```python
from build123d import *

# Parameters (mm, degrees)
SKETCH1_R               = 2.54
BOSS_EXTRUDE1_DEPTH     = 6.35
SKETCH2_R               = 2.54
BOSS_EXTRUDE2_DEPTH     = 6.35
CUT_EXTRUDE3_DEPTH      = 191.722024651
BOSS_EXTRUDE3_START     = -6.35
BOSS_EXTRUDE3_OUTLINE_R = 2.54
BOSS_EXTRUDE3_DEPTH     = 6.35


# Read off the part's stored shape, not the designer's step: Boss-Extrude3
with BuildPart() as part:
    # Sketch1 → Boss-Extrude1 (new body)
    with BuildSketch(Plane(origin=(0, 0, 0), x_dir=(0, 0, -1), z_dir=(1, 0, 0))):
        with BuildLine():
            Line((-44.569856196, 7.632792855), (2.7669164, -12.394925318))
            ThreePointArc((2.7669164, -12.394925318), (12.623500932, 1.391842028), (0, 12.7))
            ThreePointArc((0, 12.7), (-15.936201096, 21.312567622), (-17.462784388, 39.362730221))
            ThreePointArc((-17.462784388, 39.362730221), (-5.921340573, 86.302722272), (-10.695095154, 134.404479477))
            Line((-10.695095154, 134.404479477), (-17.44376381, 158.89152649))
            ThreePointArc((-17.44376381, 158.89152649), (-33.061621644, 167.760715668), (-41.930810822, 152.142857834))
            Line((-41.930810822, 152.142857834), (-38.556476494, 139.899334328))
            Line((-38.556476494, 139.899334328), (-35.182142166, 127.655810822))
            ThreePointArc((-35.182142166, 127.655810822), (-31.257188906, 88.106825725), (-40.746496905, 49.513037183))
            ThreePointArc((-40.746496905, 49.513037183), (-46.038128876, 28.881479889), (-44.569856196, 7.632792855))
        make_face()
        Circle(SKETCH1_R, mode=Mode.SUBTRACT)
        with Locations((-31.007118959, 161.740192162)):
            Circle(SKETCH1_R, mode=Mode.SUBTRACT)
    extrude(amount=BOSS_EXTRUDE1_DEPTH)

    # Sketch2 → Boss-Extrude2 (add)
    with BuildSketch(Plane(origin=(6.35, 0, 0), x_dir=(0, 0, -1), z_dir=(1, 0, 0))):
        with BuildLine():
            Line((-44.569856196, 7.632792855), (-42.095309311, -5.538639039))
            ThreePointArc((-42.095309311, -5.538639039), (-43.548594954, -20.911029153), (-52.944669407, -33.164037021))
            Line((-52.944669407, -33.164037021), (-59.696430917, -38.15584))
            Line((-59.696430917, -38.15584), (-89.652353277, -43.783727307))
            Line((-89.652353277, -43.783727307), (-86.13492371, -62.506178782))
            Line((-86.13492371, -62.506178782), (-48.69002076, -55.471319649))
            Line((-48.69002076, -55.471319649), (2.7669164, -12.394925318))
            Line((2.7669164, -12.394925318), (-44.569856196, 7.632792855))
        make_face()
        with Locations((-75.412004177, -50.8)):
            Circle(SKETCH2_R, mode=Mode.SUBTRACT)
    extrude(amount=-BOSS_EXTRUDE2_DEPTH)

    # Sketch7 → Cut-Extrude3 (cut, through all)
    with BuildSketch(Plane(origin=(6.35, 0, 0), x_dir=(0, 0, -1), z_dir=(1, 0, 0))):
        Polygon((-46.865774263, -27.0023496), (-22.96155218, -33.933122483), (78.29652169, 5.436064098), (-6.223292372, 82.704708682), (-31.505451919, 85.148559871), (-103.235957303, 48.493013889), align=None)
    extrude(amount=-CUT_EXTRUDE3_DEPTH, mode=Mode.SUBTRACT)


with BuildPart() as cut_extrude3_piece_1:
    # of the separate pieces the step leaves, piece 1, a body of its own (cut_extrude3_pieces)
    add(part.part.solids().sort_by_distance((0, 127.655810822, 35.182142166))[0])



with BuildPart() as cut_extrude3_piece_2:
    # of the separate pieces the step leaves, piece 2, a body of its own (cut_extrude3_pieces)
    add(part.part.solids().sort_by_distance((0, -27.0023496, 46.865774263))[0])


with BuildPart() as cut_extrude3_piece_1_1:
    add(cut_extrude3_piece_1.part)

    add(cut_extrude3_piece_2.part)  # Boss-Extrude3 merges Cut-Extrude3 piece 2
    # Boss-Extrude3 outline → Boss-Extrude3 (add)
    with BuildSketch(Plane(origin=(6.35, 0, 0), x_dir=(0, 0, -1), z_dir=(1, 0, 0)).offset(BOSS_EXTRUDE3_START)):
        with BuildLine():
            ThreePointArc((-17.94031666, 2.919785972), (-45.017090497, 8.492394425), (-37.839830784, 35.188697342))
            ThreePointArc((-37.839830784, 35.188697342), (-16.082022846, 54.987957012), (-6.223292372, 82.704708682))
            Line((-6.223292372, 82.704708682), (-31.505451919, 85.148559871))
            ThreePointArc((-31.505451919, 85.148559871), (-37.228581056, 69.058602906), (-49.859288922, 57.564859346))
            ThreePointArc((-49.859288922, 57.564859346), (-73.23147922, 17.433041422), (-48.0280892, -21.574793953))
            ThreePointArc((-48.0280892, -21.574793953), (-46.322848152, -24.047848471), (-46.865774263, -27.0023496))
            Line((-46.865774263, -27.0023496), (-22.96155218, -33.933122483))
            Line((-22.96155218, -33.933122483), (2.7669164, -12.394925318))
            ThreePointArc((2.7669164, -12.394925318), (11.617144077, 5.131467967), (-7.298891252, 10.393083589))
            Line((-7.298891252, 10.393083589), (-17.94031666, 2.919785972))
        make_face()
        Circle(BOSS_EXTRUDE3_OUTLINE_R, mode=Mode.SUBTRACT)
    extrude(amount=BOSS_EXTRUDE3_DEPTH)


solid = cut_extrude3_piece_1_1.part
```
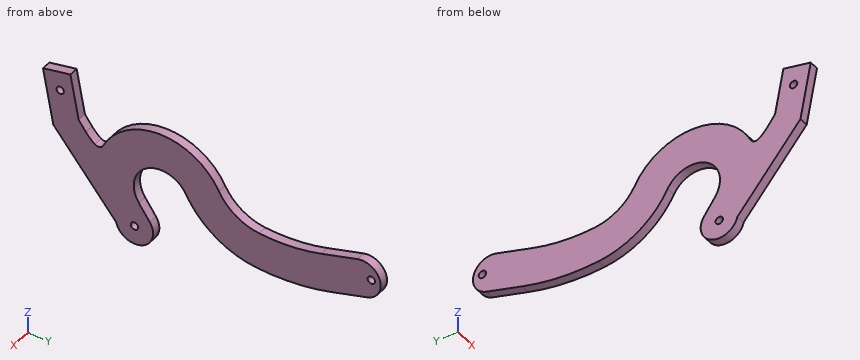
The listing builds one solid part. Answer for the finished solid, in the listing's coordinates (mm). Give positions to 0.01 mm unless a question says otherwise; leave off trailing zeros. Write each loop counter-clockwise with the first axis right and the second up, starting at its lowest first coordinate (ties: lowest second). Pieces come first, ordered by that corner, then holes. Notation, with made-up numbers: M 42.25,-22 L 48.25,-22 A26 ccw 48.25,-8 Z; hole C 33,32 d4. An arc over 180 degrees is marked long. Write each question's results on one line, items separated by ' | '.
Q1. Section B-B, the plane y = -50.8 is taken. Write down the section's boundary in (x, z).
Output values:
outline: M 0,43.11 L 6.35,43.11 L 6.35,72.87 L 0,72.87 Z; M 0,77.95 L 6.35,77.95 L 6.35,88.33 L 0,88.33 Z
Q2. Flat-ended cylindrical pins translate along their axes: P1, Ø4, axis at y = 161.74, z = 31.01, coming from the -X side; P2, Ø1.5, axis at x = 3, y = 94, coming from the -Z side; P3, Ø1, axis at x = 5.5, z = 3, coming from the +Y side. Find the tip coordinate at first contact, or state that the pin passes through.
Output values:
P1: through | P2: z = 5.57 | P3: y = 12.45
Q3. Section C-C, the plane x = 4.5 is taken. Write down the section's boundary in (y, z), then the cut area to 3 significant figures.
Output values:
outline: M -62.51,86.13 L -55.47,48.69 L -12.39,-2.77 A12.7 ccw long 10.39,7.3 L 2.92,17.94 A18.99 cw long 35.19,37.84 A60.55 ccw 82.7,6.22 A142.85 ccw 134.4,10.7 L 158.89,17.44 A12.7 ccw 152.14,41.93 L 127.66,35.18 A117.45 cw 85.15,31.51 A35.15 cw 57.56,49.86 A44.39 ccw -21.57,48.03 A3.92 cw -27,46.87 A27.94 cw -33.16,52.94 L -38.16,59.7 L -43.78,89.65 Z; hole C -50.8,75.41 d5.08; hole C 0,0 d5.08; hole C 161.74,31.01 d5.08 | area: 7,800 mm2
Q4. Section D-D, the plane y = 125.5 is taken. Write down the section's boundary in (x, z).
Output values:
outline: M 0,8.55 L 6.35,8.55 L 6.35,34.61 L 0,34.61 Z
Q5. Consider L1, parallel to Y at x = 5.25, z = 66; L2, parallel to Z at x = 4.5, y = 96; L3, parallel to Y at x = 5.75, z = 18. Determine where each line is inside the solid, lowest interval first. Write a range as from..to.
Output values:
L1: -58.72..-39.34, -5.84..42.76 | L2: 5.56..30.96 | L3: -29.78..2.88, 52.27..160.49
Q6. Section A-A, the plane z = 63 is taken. Write down the section's boundary in (x, y).
Output values:
outline: M 0,-58.16 L 6.35,-58.16 L 6.35,-38.78 L 0,-38.78 Z; M 0,-9.9 L 6.35,-9.9 L 6.35,46.82 L 0,46.82 Z
